from build123d import *

# Parameters (mm, degrees)
CROQUIS1_R                 = 5
SALIENTE_EXTRUIR1_DEPTH    = 12.5
CROQUIS2_R                 = 2
CORTAR_EXTRUIR1_DEPTH      = 15.5
CROQUIS3_R                 = 2
CORTAR_EXTRUIR2_DEPTH      = 2.5
CROQUIS4_R                 = 4
SALIENTE_EXTRUIR2_DEPTH    = 15
CROQUIS5_W                 = 5.65685425
CROQUIS5_H                 = 5.65685425
SALIENTE_EXTRUIR3_DEPTH    = 10
CORTAR_EXTRUIR3_REACH      = 40.568
CORTAR_EXTRUIR3_END_RADIUS = 2
CROQUIS6_R                 = 1.265
CROQUIS7_W                 = 4
CROQUIS7_H                 = 10
CORTAR_EXTRUIR4_DEPTH      = 2
CROQUIS8_R                 = 2.5
SALIENTE_EXTRUIR4_DEPTH    = 100


with BuildPart() as part:
    # Croquis1 → Saliente-Extruir1 (new, symmetric)
    with BuildSketch(Plane.XY):
        Circle(CROQUIS1_R)
    extrude(amount=SALIENTE_EXTRUIR1_DEPTH, both=True)

    # Croquis2 → Cortar-Extruir1 (cut)
    with BuildSketch(Plane(origin=(0, 0, -12.5), x_dir=(-1, 0, 0), z_dir=(0, 0, -1))):
        Circle(CROQUIS2_R)
    extrude(amount=-CORTAR_EXTRUIR1_DEPTH, mode=Mode.SUBTRACT)

    # Croquis3 → Cortar-Extruir2 (cut)
    with BuildSketch(Plane(origin=(0, 5, 0), x_dir=(1, 0, 0), z_dir=(0, 1, 0))):
        with Locations(Location((0, 4.5, 0), (0, 0, 270))):
            Circle(CROQUIS3_R)
    extrude(amount=-CORTAR_EXTRUIR2_DEPTH, mode=Mode.SUBTRACT)

    # Croquis4 → Saliente-Extruir2 (add)
    with BuildSketch(Plane.XY.offset(12.5)):
        Circle(CROQUIS4_R)
    extrude(amount=SALIENTE_EXTRUIR2_DEPTH)

    # Croquis5 → Saliente-Extruir3 (add)
    with BuildSketch(Plane.XY.offset(27.5)):
        Rectangle(CROQUIS5_W, CROQUIS5_H)
    extrude(amount=SALIENTE_EXTRUIR3_DEPTH)

    # Cortar-Extruir3: up to this cylinder (the profile starts outside it)
    cortar_extruir3_end = Plane(origin=(0, 0, -4.5), z_dir=(0, 0, -1)) * Cylinder(CORTAR_EXTRUIR3_END_RADIUS, 86.136, mode=Mode.PRIVATE)
    # Croquis6 → Cortar-Extruir3 (cut, up to the surface)
    with BuildSketch(Plane(origin=(0, 2.5, 0), x_dir=(1, 0, 0), z_dir=(0, 1, 0)), mode=Mode.PRIVATE) as cortar_extruir3_sk1:
        with Locations(Location((0, 4.5, 0), (0, 0, 270))):
            Circle(CROQUIS6_R)
    cortar_extruir3_tool1 = extrude(cortar_extruir3_sk1.sketch, amount=-CORTAR_EXTRUIR3_REACH, mode=Mode.PRIVATE) - cortar_extruir3_end
    add(cortar_extruir3_tool1.solids().sort_by_distance((0, 2.5, -4.5))[0], mode=Mode.SUBTRACT)

    # Croquis7 → Cortar-Extruir4 (cut)
    with BuildSketch(Plane(origin=(0, -5, 0), x_dir=(-1, 0, 0), z_dir=(0, -1, 0))):
        Rectangle(CROQUIS7_W, CROQUIS7_H)
    extrude(amount=-CORTAR_EXTRUIR4_DEPTH, mode=Mode.SUBTRACT)

    # Croquis8 → Saliente-Extruir4 (add)
    with BuildSketch(Plane.XY.offset(37.5)):
        Circle(CROQUIS8_R)
    extrude(amount=SALIENTE_EXTRUIR4_DEPTH)


solid = part.part
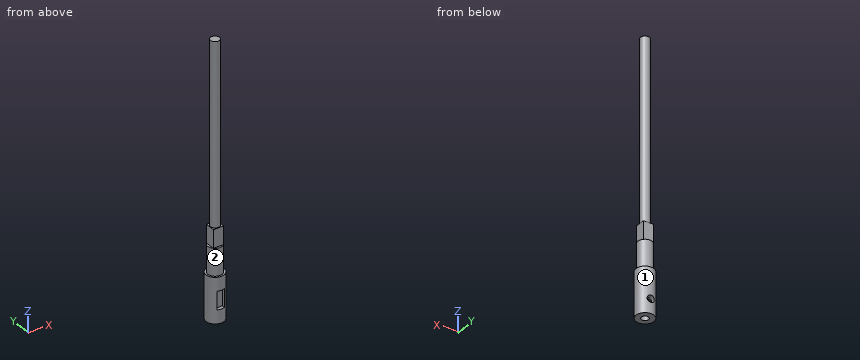
Geometry check sheet. Reference: the model listing, model coordinates, mm. Face numbers are marked on the shaded views. A direction names the side the tool comes from. Give positions to 0.01 mm unless a question says otherwise; leave off trailing zeros. Order: outer loops, then holes, each group sorted by start corner. A loop starts at its lowest first (then second) coordinate and runs counter-clockwise, first axis right, second up. Notation, with made-up numbers: M 43.5,54 L 71.5,54 A16 ccw 71.5,82 Z; hole C 86.5,35 d4. An arc over 180 degrees is marked long. Use a Markdown table: item, result.
Item 1: Material ranges on line 1 along Y through (x, z) = (0, -1.25); line 2 along Z through (x, y) = (0, 2.35) (3 decimals); line 3 along Z through (x, y) = (-1.5, -3.5), recorded low to high.
Answers follow:
| item | result |
|---|---|
| line 1 | y = -3 to -2, 2 to 5 |
| line 2 | z = -12.5 to -5.765, -3.235 to 137.5 |
| line 3 | z = -12.5 to -5, 5 to 27.5 |
Item 2: Section check B-B (y = 0). Record the cut outline in (x, z), and give its area (3 significant figures).
Answers follow:
| item | result |
|---|---|
| outline | M -5,-12.5 L -2,-12.5 L -2,3 L 2,3 L 2,-12.5 L 5,-12.5 L 5,12.5 L 4,12.5 L 4,27.5 L 2.83,27.5 L 2.83,37.5 L 2.5,37.5 L 2.5,137.5 L -2.5,137.5 L -2.5,37.5 L -2.83,37.5 L -2.83,27.5 L -4,27.5 L -4,12.5 L -5,12.5 Z |
| area | 865 mm2 |
Item 3: Section check D-D (z = 112.5). Record the cut outline in (x, y), and give its area (3 significant figures).
Answers follow:
| item | result |
|---|---|
| outline | C 0,0 d5 |
| area | 19.6 mm2 |
Item 4: Depth check by flat-ended pin: P1, Ø2, axis at x = 0, z = 72, coming from the +Y side; P2, Ø2, axis at x = -3, z = 76, coming from the -Y side; P3, Ø1.3, axis at y = -3.5, z = 2, coming from the +X side. Enter the tip coordinate at first touch or a pass-through.
Answers follow:
| item | result |
|---|---|
| P1 | stops at y = 2.5 |
| P2 | stops at y = -1.5 |
| P3 | stops at x = 4.11 |
Item 5: Tool access check on the marked faces 1 and 2. Record the directions out of +Z, -Z, +X, -X, +Y, -Y that give a thin tool (end or side, any length) a straight path to the whole face; none if there is none.
Answers follow:
| item | result |
|---|---|
| face 1 | +Z, -Z |
| face 2 | +Z |
Item 6: Section check C-C (z = 35). Record the cut outline in (x, y), and give its area (3 significant figures).
Answers follow:
| item | result |
|---|---|
| outline | M -2.83,-2.83 L 2.83,-2.83 L 2.83,2.83 L -2.83,2.83 Z |
| area | 32.0 mm2 |
